```python
from build123d import *

# Parameters (mm, degrees)
SKETCH1_W           = 20.29
SKETCH1_H           = 26.42
BOSS_EXTRUDE1_DEPTH = 5.21
SKETCH2_R           = 0.915
SKETCH2_R_2         = 0.865
SKETCH2_R_3         = 0.7
BOSS_EXTRUDE2_DEPTH = 3


with BuildPart() as part:
    # Sketch1 → Boss-Extrude1 (new body)
    with BuildSketch(Plane(origin=(0, 0, 0), x_dir=(0, 0, -1), z_dir=(1, 0, 0))):
        Rectangle(SKETCH1_W, SKETCH1_H)
    extrude(amount=BOSS_EXTRUDE1_DEPTH)

    # Sketch2 → Boss-Extrude2 (add)
    with BuildSketch(Plane.XZ.offset(13.21)):
        with Locations(Location((2.605, -7.073929595, 0), (0, 0, 90))):
            Circle(SKETCH2_R)
        with Locations(Location((2.605, -3.263929595, 0), (0, 0, 90))):
            Circle(SKETCH2_R_2)
        with Locations(Location((2.605, 8.166070405, 0), (0, 0, 90))):
            Circle(SKETCH2_R_3)
    extrude(amount=BOSS_EXTRUDE2_DEPTH)


solid = part.part
```
Check sheet for the modelled part. Datum: model origin and axes. Units: mm. A direction names the side the tool comes from. Round coordinates to 2 decimals unless told otherwise and drop trailing zeros. Order: outer loops, then holes, each group sorted by start corner. A loop starts at its lowest first (then second) coordinate and runs counter-clockwise, first axis right, second up.
1) Scan line: line 1 (Y direction, x = 3.5, z = 4.75). Record every from-to range of solid material in increasing order.
2) Tool access check on faces 1 (the flat face through (0, 0, 0)), 2 (the cylindrical face through (2.9, -14.7, 8.8)). Record the directions out of +Z, -Z, +X, -X, +Y, -Y that give a thin tool (end or side, any length) a straight path to the whole face; none if there is none.
3) Section check D-D (x = 4.2). Record the boundary of the cut face in (y, z) (3 decimals), and give its area (3 significant figures).
4) Section check C-C (y = -13.75). Record the boundary of the cut face in (x, z) (3 decimals).
5) Section check A-A (x = 2.2). Record the boundary of the cut face in (y, z) (3 decimals), and give its area (3 significant figures).
6) Mould release check, pull along Z, two halves, no side actions. Record for faces 3 (the flat face through (3, 0, -10.145)), 4 (the flat face through (3, -13.21, 0)), 5 (the flat face through (3, -16.21, -7)), 6 (the cylindrical face through (2.565, -14.689, -7.988)): +Z half, -Z half, draft (parallel to the pull), parting line (faces both ways), or undercut.
7) Go/stop test with a flat-tipped pin: pin 1 Ø1.5 at (x, z) = (2.5, 4.5) entering from -Y. Record where the tip stops, or that it passes through.
8) Section check B-B (z = -0.25). Record the boundary of the cut face in (x, y), and give its area (3 significant figures).
Result:
1. line 1: y = -13.21 to 13.21
2. face 1: +Z, -Z, -X, +Y, -Y
2. face 2: -Y
3. outline: (-13.21, -10.145) - (13.21, -10.145) - (13.21, 10.145) - (-13.21, 10.145) - close
3. area: 536 mm2
4. outline: circle Ø1.83 at (2.605, -7.074); circle Ø1.73 at (2.605, -3.264); circle Ø1.4 at (2.605, 8.166)
5. outline: (-16.21, -7.894) - (-13.21, -7.894) - (-13.21, -10.145) - (13.21, -10.145) - (13.21, 10.145) - (-13.21, 10.145) - (-13.21, 8.737) - (-16.21, 8.737) - (-16.21, 7.595) - (-13.21, 7.595) - (-13.21, -2.5) - (-16.21, -2.5) - (-16.21, -4.028) - (-13.21, -4.028) - (-13.21, -6.253) - (-16.21, -6.253) - close
5. area: 549 mm2
6. face 3: -Z half
6. face 4: undercut
6. face 5: draft
6. face 6: undercut
7. pin 1: stops at y = -13.21
8. outline: (0, -13.21) - (5.21, -13.21) - (5.21, 13.21) - (0, 13.21) - close
8. area: 138 mm2
